Design review of the part shown in the three views and the two pictorial views. Dimensions are in mm from the part's minimum x, y and z. A direction names the side the tool comes from. Round coordinates to 2 decimals unless told otherwise and drop trailing zeros. Write each loop counter-clockwise with the first axis right and the second up, starting at its lowest first coordinate (ties: lowest second). Pieces come first, ordered by that corner, then holes. Notation, with made-up numbers: (17.5, -38.75) - (55.5, -38.75) arc R18 ccw to (55.5, -31.75) - close; hole circle Ø6 at (6.5, 0.25). An arc over 180 degrees is marked (long way). Use one line per item in the form item = value.
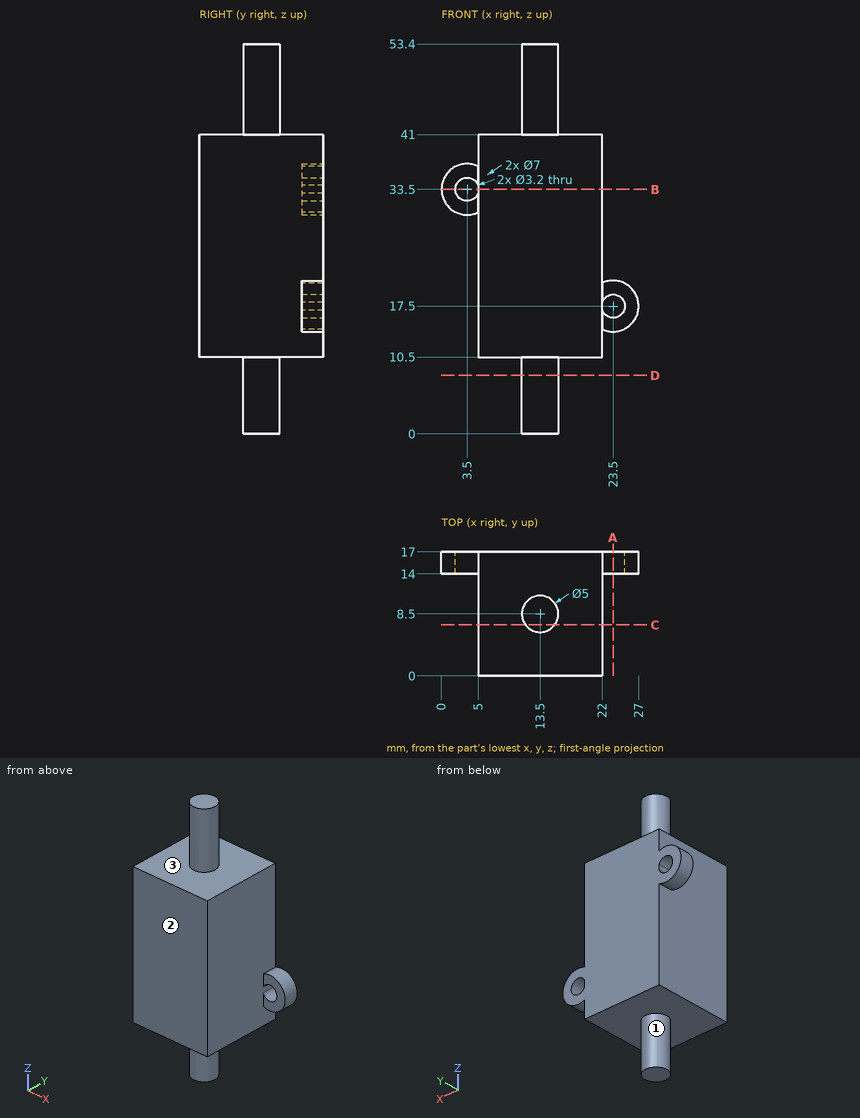
(1) Insertion check: P1, Ø2, axis at y = 5.5, z = 9, coming from the +X side; P2, Ø1.5, axis at x = 1.5, z = 32, coming from the -Y side; P3, Ø4, axis at x = 5.5, y = 15, coming from the -Z side; P4, Ø2.5, axis at x = 23.5, z = 17.5, coming from the +Y side. Each pin has a flat end and moves straight along its axis. Give the tip position at first contact, or say it passes through.
Geometry results:
P1 = 15
P2 = 14
P3 = 10.5
P4 = through
(2) Add section D-D on z = 8. Write out the cut boundary in (x, y).
Geometry results:
outline = circle Ø5 at (13.5, 8.5)
(3) To check wall thickness, follow L1, parallel to Z at x = 3.5, y = 15.6; L2, parallel to X at y = 14.8, z = 17.5; L3, parallel to X at y = 6.5, z = 17.5. State the ranges of each line that lie inside material, in increasing order.
Geometry results:
L1 = 30 to 31.9, 35.1 to 37
L2 = 5 to 22, 25.1 to 27
L3 = 5 to 22
(4) Add section B-B on z = 33.5. Write out the cut boundary in (x, y).
Geometry results:
outline = (0, 14) - (1.9, 14) - (1.9, 17) - (0, 17) - close; (5, 0) - (22, 0) - (22, 17) - (5, 17) - close
(5) Machinability: for the marked faces 1, 2 and 3, which of the approach directions +Z, -Z, +X, -X, +Y, -Y give a long, thin tool a straight path to every point of the face, cutting with its end or side? Answer none if there is none.
Geometry results:
face_1 = -Z
face_2 = +Z, -Z, +X, -X, -Y
face_3 = +Z
(6) Add section A-A on x = 23.5. Write out the cut boundary in (y, z), then the cut area to 3 significant figures.
Geometry results:
outline = (14, 14) - (17, 14) - (17, 15.9) - (14, 15.9) - close; (14, 19.1) - (17, 19.1) - (17, 21) - (14, 21) - close
area = 11.4 mm2
(7) Add section C-C on y = 7. Write out the cut boundary in (x, z).
Geometry results:
outline = (5, 10.5) - (11.5, 10.5) - (11.5, 0) - (15.5, 0) - (15.5, 10.5) - (22, 10.5) - (22, 41) - (15.5, 41) - (15.5, 53.4) - (11.5, 53.4) - (11.5, 41) - (5, 41) - close
